Geometry: see drawing. Coordinates: mm, zero at the bounding-box minimum. Coordinates: 2 decimals unless noted, no trailing zeros. Write each loop counter-clockwise with the first axis right and the second up, starting at its lowest first coordinate (ties: lowest second). Pieces come first, ordered by that corner, then holes. Notation, with made-up numbers: (76.25, 65) - (106.25, 65) arc R34 cw to (106.25, 100) - close; hole circle Ø7 at (-2.5, 41.5). An arc over 180 degrees is marked (long way). Use a Markdown table: item, result. Add a question column.
Q1. Section query A-A (x = 82). Return the cut outline in (y, z), then the cut area to 3 significant figures.
Q2. Section query C-C (y = 85). Return the cut outline in (x, z), then the cut area to 3 significant figures.
Q3. Pin query (flat end, axial travel): P1, Ø11, axis at x = 15.25, y = 85, coming from the -Z side (3 decimals). Return the tip coordinate at first contact, or that it passes through.
Q4. Material intervals for probe 1 along Y at (x, z) = (82, 1.4); probe 2 along X at (y, z) = (87.5, 4.1); probe 3 along Y at (x, z) = (148.75, 3.65), sorted ascending. Write a range as from..to.
Q5. Section query B-B (y = 125). Return the cut outline in (x, z), then the cut area to 3 significant figures.
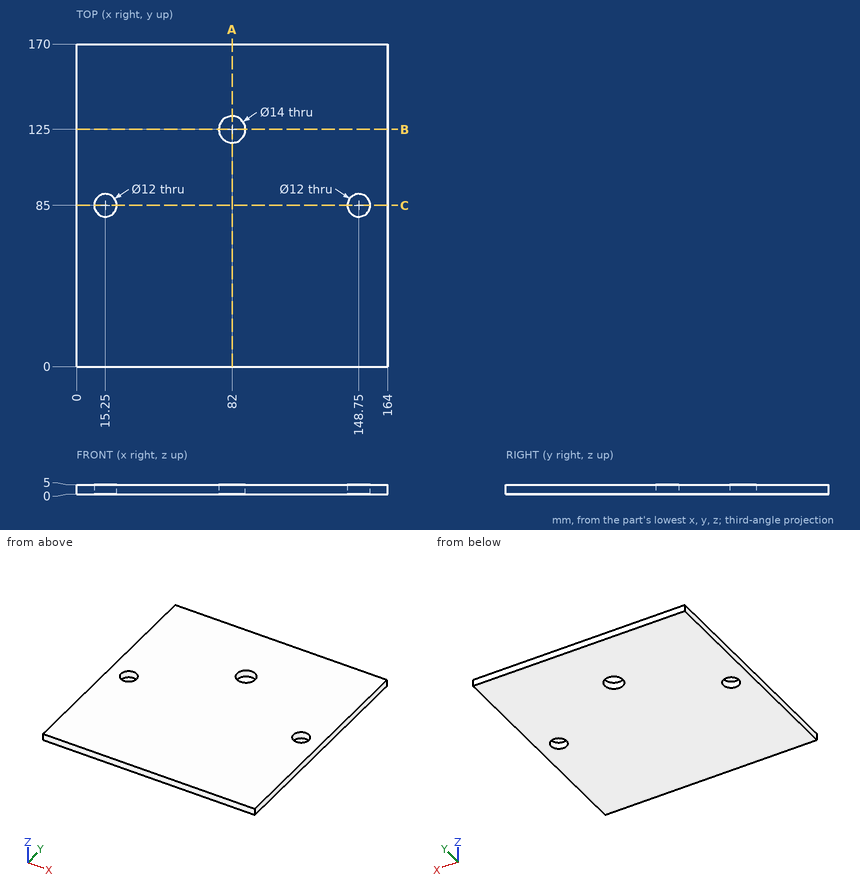
Values follow:
| question | item | result |
|---|---|---|
| 1 | outline | (0, 0) - (118, 0) - (118, 5) - (0, 5) - close; (132, 0) - (170, 0) - (170, 5) - (132, 5) - close |
| 1 | area | 780 mm2 |
| 2 | outline | (0, 0) - (9.25, 0) - (9.25, 5) - (0, 5) - close; (21.25, 0) - (142.75, 0) - (142.75, 5) - (21.25, 5) - close; (154.75, 0) - (164, 0) - (164, 5) - (154.75, 5) - close |
| 2 | area | 700 mm2 |
| 3 | P1 | through |
| 4 | probe 1 | 0..118, 132..170 |
| 4 | probe 2 | 0..9.8, 20.7..143.3, 154.2..164 |
| 4 | probe 3 | 0..79, 91..170 |
| 5 | outline | (0, 0) - (75, 0) - (75, 5) - (0, 5) - close; (89, 0) - (164, 0) - (164, 5) - (89, 5) - close |
| 5 | area | 750 mm2 |
